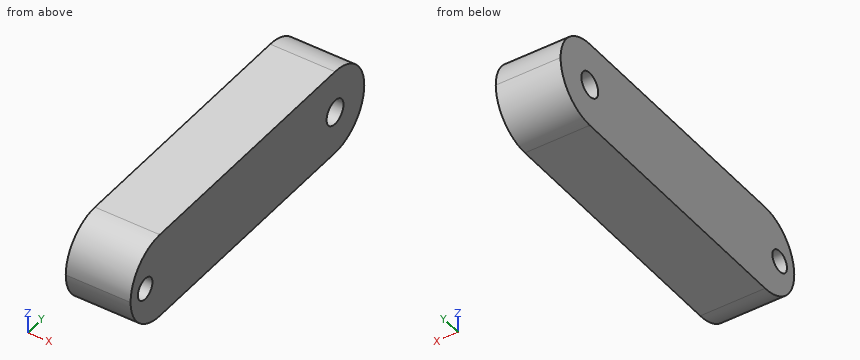
```python
from build123d import *

# Parameters (mm, degrees)
SKETCH1_W           = 38.1
SKETCH1_H           = 50.8
BOSS_EXTRUDE1_DEPTH = 101.6
SKETCH2_R           = 6.35
CUT_EXTRUDE1_DEPTH  = 112.44204772
FILLET1_R           = 25.4
SKETCH3_R           = 7.332348419
CUT_EXTRUDE2_DEPTH  = 441.771925846


with BuildPart() as part:
    # Sketch1 → Boss-Extrude1 (new, symmetric)
    with BuildSketch(Plane(origin=(0, 0, 0), x_dir=(1, 0, 0), z_dir=(0, 1, 0))):
        Rectangle(SKETCH1_W, SKETCH1_H)
    extrude(amount=BOSS_EXTRUDE1_DEPTH, both=True)

    # Sketch2 → Cut-Extrude1 (cut, through all)
    with BuildSketch(Plane(origin=(19.05, 0, 0), x_dir=(0, 0, -1), z_dir=(1, 0, 0))):
        with Locations((0, -88.9)):
            Circle(SKETCH2_R)
    extrude(amount=-CUT_EXTRUDE1_DEPTH, mode=Mode.SUBTRACT)

    # Fillet1
    fillet1_edges = [part.edges().sort_by_distance(p)[0] for p in [
        (0, -101.6, -25.4),
        (0, -101.6, 25.4),
        (0, 101.6, 25.4),
        (0, 101.6, -25.4),
    ]]
    fillet(fillet1_edges, radius=FILLET1_R - 0.0001)  # a hair under: the kernel refuses the full size

    # Sketch3 → Cut-Extrude2 (cut, through all)
    with BuildSketch(Plane(origin=(292.1, -73.474884434, -233.084724799), x_dir=(0, 0.5719099585576003, -0.8203164019466171), z_dir=(1, 0, 0))):
        with Locations(Location((-105.602665842, 256.084237961, 0), (0, 0, 325.116479352))):
            Circle(SKETCH3_R)
    extrude(amount=-CUT_EXTRUDE2_DEPTH, mode=Mode.SUBTRACT)


solid = part.part
```
Design review of the part built by this model. Coordinates are the model's own, in mm. Give positions to 0.01 mm unless a question says otherwise; leave off trailing zeros. Write each loop counter-clockwise with the first axis right and the second up, starting at its lowest first coordinate (ties: lowest second). Pieces come first, ordered by that corner, then holes. Notation, with made-up numbers: (19, 28.5) -> (59, 28.5) arc R13 cw to (59, 49.5) -> close; hole circle Ø11 at (-9, 62.25). An arc over 180 degrees is marked (long way). Answer in a Markdown table with one row per item.
(1) To check wall thickness, follow probe 1 along Y at (x, z) = (8, 0); probe 2 along Z at (x, y) = (-16, -86); probe 3 along Z at (x, y) = (4, -88). State the ranges of each line that lie inside material, in increasing order.
Results:
| item | result |
|---|---|
| probe 1 | -101.6 to -95.25, -82.55 to 68.87, 83.53 to 101.6 |
| probe 2 | -23.43 to -5.65, 5.65 to 23.43 |
| probe 3 | -22.49 to -6.29, 6.29 to 22.49 |
(2) Clearance check with flat-ended pins moving along their axes: pin 1 (1 mm diameter, centred on x = 10, z = -2, fed in from -Y); pin 2 (1.5 mm diameter, centred on x = -6.5, z = 10, fed in from -Y). State where each tip first meets the part, or that it passes through.
Results:
| item | result |
|---|---|
| pin 1 | y = -101.56 |
| pin 2 | y = -99.86 |
(3) Consider section B-B (y = -88.9). State the section outline as (x, z) points.
Results:
| item | result |
|---|---|
| outline | (-19.05, -22) -> (19.05, -22) -> (19.05, -6.35) -> (-19.05, -6.35) -> close; (-19.05, 6.35) -> (19.05, 6.35) -> (19.05, 22) -> (-19.05, 22) -> close |
(4) Consider section D-D (z = 12.5). State the section outline as (x, y) points.
Results:
| item | result |
|---|---|
| outline | (-19.05, -98.31) -> (19.05, -98.31) -> (19.05, 98.31) -> (-19.05, 98.31) -> close |
(5) Consider section C-C (z = -20). State the section outline as (x, y) points, then the cut area to 3 significant figures.
Results:
| item | result |
|---|---|
| outline | (-19.05, -91.86) -> (19.05, -91.86) -> (19.05, 91.86) -> (-19.05, 91.86) -> close |
| area | 7,000 mm2 |
(6) Consider section A-A (x = 16.5). Count the separate pieces of the cut face and the enclosed holes in it, then the cut area to 3 significant figures.
Results:
| item | result |
|---|---|
| separate pieces | 1 |
| enclosed holes | 2 |
| area | 9,470 mm2 |
